```python
from build123d import *

# Parameters (mm, degrees)
CROQUIS1_R                                  = 2
CROQUIS1_W                                  = 7
CROQUIS1_H                                  = 58
SALIENTE_EXTRUIR1_DEPTH                     = 1
AVELLANADO_PARA_TORNILLO_CON_CABEZA_2_COUNT = 2
AVELLANADO_PARA_TORNILLO_CON_CABEZA_2_PITCH = 70


with BuildPart() as part:
    # Croquis1 → Saliente-Extruir1 (new body)
    with BuildSketch(Plane.XY):
        with BuildLine():
            Line((-11, 36), (-11, -36))
            ThreePointArc((-11, -36), (-9.828427125, -38.828427125), (-7, -40))
            Line((-7, -40), (7, -40))
            ThreePointArc((7, -40), (9.828427125, -38.828427125), (11, -36))
            Line((11, -36), (11, 36))
            ThreePointArc((11, 36), (9.828427125, 38.828427125), (7, 40))
            Line((7, 40), (-7, 40))
            ThreePointArc((-7, 40), (-9.828427125, 38.828427125), (-11, 36))
        make_face()
        with Locations((0, 35)):
            Circle(CROQUIS1_R, mode=Mode.SUBTRACT)
        with Locations((0, -35)):
            Circle(CROQUIS1_R, mode=Mode.SUBTRACT)
        with Locations((4.5, 0)):
            Rectangle(CROQUIS1_W, CROQUIS1_H, mode=Mode.SUBTRACT)
    extrude(amount=SALIENTE_EXTRUIR1_DEPTH)

    # Croquis6 → Avellanado para tornillo con cabeza elevada avellanada de M41 (revolve, cut)
    with BuildSketch(Plane(origin=(0, 35, 1), x_dir=(0, -1, 0), z_dir=(1, 0, 0))):
        Polygon((0, 0), (0, 1), (2.25, 1), (2.25, 0.75), (3, 0), align=None)
    avellanado_para_tornillo_con_cabeza_elev = revolve(axis=Axis((0, 35, 7.35), (0, 0, -1)), mode=Mode.SUBTRACT)

    # Avellanado para tornillo con cabeza  2: Avellanado para tornillo con cabeza elevada avellanada de M41 ×2
    with Locations(*[(0, -i * AVELLANADO_PARA_TORNILLO_CON_CABEZA_2_PITCH, 0) for i in range(1, AVELLANADO_PARA_TORNILLO_CON_CABEZA_2_COUNT)]):
        add(avellanado_para_tornillo_con_cabeza_elev, mode=Mode.SUBTRACT)


solid = part.part
```
Check sheet for the modelled part. Datum: model origin and axes. Units: mm. Coordinates: 2 decimals unless noted, no trailing zeros. Loops run counter-clockwise (first coordinate to the right, second up) from the corner with the lowest first, then second, coordinate; pieces in that order, holes last.
1) Sectioned sample at D-D (z = 0.6). Record the boundary of the cut face in (x, y).
2) Sectioned sample at C-C (x = 4.75). Record the boundary of the cut face in (y, z).
3) Material ranges on probe 1 along Y at (x, z) = (0, 0.25); probe 2 along X at (y, z) = (35, 0.1), recorded low to high.
4) Sectioned sample at B-B (x = 0). Record the boundary of the cut face in (y, z).
5) Sectioned sample at A-A (y = 35). Record the boundary of the cut face in (x, z), and give its area (3 significant figures).
Check sheet entries:
1. outline: (-11, -36) arc R4 ccw to (-7, -40) - (7, -40) arc R4 ccw to (11, -36) - (11, 36) arc R4 ccw to (7, 40) - (-7, 40) arc R4 ccw to (-11, 36) - close; hole circle Ø5.2 at (0, -35); hole circle Ø5.2 at (0, 35); hole (1, -29) - (8, -29) - (8, 29) - (1, 29) - close
2. outline: (-40, 0) - (-29, 0) - (-29, 1) - (-40, 1) - close; (29, 0) - (40, 0) - (40, 1) - (29, 1) - close
3. probe 1: y = -40 to -37.25, -32.75 to 32.75, 37.25 to 40
3. probe 2: x = -11 to -2.25, 2.25 to 11
4. outline: (-40, 0) - (-37.25, 0) - (-37.25, 0.25) - (-38, 1) - (-40, 1) - close; (-32.75, 0) - (32.75, 0) - (32.75, 0.25) - (32, 1) - (-32, 1) - (-32.75, 0.25) - close; (37.25, 0) - (40, 0) - (40, 1) - (38, 1) - (37.25, 0.25) - close
5. outline: (-11, 0) - (-2.25, 0) - (-2.25, 0.25) - (-3, 1) - (-11, 1) - close; (2.25, 0) - (11, 0) - (11, 1) - (3, 1) - (2.25, 0.25) - close
5. area: 16.9 mm2
